```python
from build123d import *

# Parameters (mm, degrees)
BOSS_EXTRUDE1_DEPTH = 19.05
CUT_EXTRUDE1_DEPTH  = 20.05
CIRPATTERN1_COUNT   = 4


with BuildPart() as part:
    # Sketch1 → Boss-Extrude1 (new body)
    with BuildSketch(Plane(origin=(0, 0, 0), x_dir=(1, 0, 0), z_dir=(0, 1, 0))):
        Polygon((-50.8, -21.042048969), (-50.8, 21.042048969), (-21.042048969, 50.8), (21.042048969, 50.8), (50.8, 21.042048969), (50.8, -21.042048969), (21.042048969, -50.8), (-21.042048969, -50.8), align=None)
        Polygon((-25.4, 10.521024484), (-10.521024484, 25.4), (10.521024484, 25.4), (25.4, 10.521024484), (25.4, -10.521024484), (10.521024484, -25.4), (-10.521024484, -25.4), (-25.4, -10.521024484), align=None, mode=Mode.SUBTRACT)
    extrude(amount=BOSS_EXTRUDE1_DEPTH)

    # Sketch2 → Cut-Extrude1 (cut, through all)
    with BuildSketch(Plane(origin=(0, 19.05, 0), x_dir=(1, 0, 0), z_dir=(0, 1, 0))):
        with BuildLine():
            Line((33.3375, 12.7), (42.8625, 12.7))
            ThreePointArc((42.8625, 12.7), (45.10756403, 11.77006403), (46.0375, 9.525))
            Line((46.0375, 9.525), (46.0375, -9.525))
            ThreePointArc((46.0375, -9.525), (45.10756403, -11.77006403), (42.8625, -12.7))
            Line((42.8625, -12.7), (33.3375, -12.7))
            ThreePointArc((33.3375, -12.7), (31.09243597, -11.77006403), (30.1625, -9.525))
            Line((30.1625, -9.525), (30.1625, 9.525))
            ThreePointArc((30.1625, 9.525), (31.09243597, 11.77006403), (33.3375, 12.7))
        make_face()
    cut_extrude1 = extrude(amount=-CUT_EXTRUDE1_DEPTH, mode=Mode.SUBTRACT)

    # Sketch4 → 1_2 Clearance Hole1 (revolve, cut)
    with BuildSketch(Plane(origin=(50.8, 9.525, 0), x_dir=(0, 0, -1), z_dir=(0, 1, 0))):
        Polygon((0, 0), (0, 67.553549943), (6.74624, 63.5), (6.74624, 0), align=None)
    f_1_2_clearance_hole1 = revolve(axis=Axis((57.15, 9.525, 0), (-1, 0, 0)), mode=Mode.SUBTRACT)

    # CirPattern1: Cut-Extrude1, 1_2 Clearance Hole1 ×4 about axis
    cirpattern1_axis = Axis((0, 0, 0), (0, 1, 0))
    for i in range(1, CIRPATTERN1_COUNT):
        add(cut_extrude1.rotate(cirpattern1_axis, i * 360 / CIRPATTERN1_COUNT), mode=Mode.SUBTRACT)
        add(f_1_2_clearance_hole1.rotate(cirpattern1_axis, i * 360 / CIRPATTERN1_COUNT), mode=Mode.SUBTRACT)


solid = part.part
```
For this review, take the finished solid that the model builds, in its own axes (mm). A direction names the side the tool comes from. Give positions to 0.01 mm unless a question says otherwise; leave off trailing zeros. Write each loop counter-clockwise with the first axis right and the second up, starting at its lowest first coordinate (ties: lowest second). Pieces come first, ordered by that corner, then holes.
Item 1: The part is to be moulded in two halves that separate along Z. For faces 3 (the face through (-26, 0, 4)), 4 (the face through (4, 16, -30.162)), 5 (the face through (-36.13, 9.39, -35.71)), say which applies: +Z half, -Z half, draft (parallel to the pull), parting line (faces both ways), or undercut.
Item 2: Wall thickness on probe 1 along Z at (x, y) = (8.5, 8.75); probe 2 along X at (y, z) = (16.25, 11); probe 3 along Y at (x, z) = (0, -28.15): over which ranges is each line inside the solid? List them lowest first.
Item 3: Take a section at D-D (x = -24). Give the boundary of the cut face in (y, z).
Item 4: Insertion check: P1, Ø3, axis at x = -27.5, y = 14.5, coming from the -Z side; P2, Ø10.5, axis at y = 7.5, z = 37.5, coming from the -X side; P3, Ø10.5, axis at y = 5, z = 36.5, coming from the +X side. Each pin has a flat end and moves straight along its axis. Give the tip position at first contact, or say it passes through.
Item 5: Take a section at C-C (z = -40). Give the boundary of the cut face in (x, y), and give its area (3 significant figures).
Item 6: Machinability: for faces 1 (the face through (11.795, 9.658, -31.117)), 2 (the face through (48.45, 16.11, 1.46)), which of the approach directions +Z, -Z, +X, -X, +Y, -Y give a long, thin tool a straight path to every point of the face, cutting with its end or side? Answer none if there is none.
Item 7: Take a section at A-A (z = 0). Give the number of separate pieces and of enclosed holes in the cut face, and give its area (3 significant figures).
Established:
1. face 3: draft
1. face 4: undercut
1. face 5: -Z half
2. probe 1: z = -50.8 to -46.04, -30.16 to -25.4, 25.4 to 30.16, 46.04 to 50.8
2. probe 2: x = -50.8 to -45.67, -30.53 to -24.92, 24.92 to 30.53, 45.67 to 50.8
2. probe 3: y = 0 to 2.78, 16.27 to 19.05
3. outline: (0, -47.84) - (19.05, -47.84) - (19.05, -11.92) - (0, -11.92) - close; (0, 11.92) - (19.05, 11.92) - (19.05, 47.84) - (0, 47.84) - close
4. P1: stops at z = -45.84
4. P2: stops at x = -39.59
4. P3: stops at x = 40.59
5. outline: (-31.84, 0) - (-12.7, 0) - (-12.7, 19.05) - (-31.84, 19.05) - close; (12.7, 0) - (31.84, 0) - (31.84, 19.05) - (12.7, 19.05) - close
5. area: 729 mm2
6. face 1: +Y, -Y
6. face 2: +X, -X
7. separate pieces: 8
7. enclosed holes: 0
7. area: 106 mm2
